Autodesk Inventor part; units mm, degrees
ref_plane "YZ Plane" through (0, 0, 0) normal (1, 0, 0) x (0, 1, 0)
ref_plane "XZ Plane" through (0, 0, 0) normal (0, 1, 0) x (-1, 0, 0)
ref_plane "XY Plane" through (0, 0, 0) normal (0, 0, 1) x (1, 0, 0)
sketch "草圖1" plane through (0, 0, 0) normal (0, 1, 0) x (-1, 0, 0)
  line L0 (0, 0) -> (-20, 0)
  line L1 (-20, 0) -> (-20, -30)
  line L2 (-20, -30) -> (0, -30)
  line L3 (0, -30) -> (0, 0)
  line L4 (-20, -30) -> (-60, -30)
  line L5 (-60, -30) -> (-60, 10)
  line L6 (-60, 10) -> (-20, 10)
  line L7 (-20, 10) -> (-20, -30)
  dimension "d0" = 20
  dimension "d1" = 40
  dimension "d2" = 40
  dimension "d3" = 30
extrude "擠出1" add sketch "草圖1" along normal blind 10
chamfer "倒角1" distance 30 distance2 40 1 edges at (60, 5, 10) measured on face at (33.3333, 3.3333, 10)
sketch "草圖2" plane through (0, 0, -30) normal (-1, 0, 0) x (0, 0, 1)
  line L0 (0, 0) -> (0, 10)
  line L1 (0, 10) -> (20, 10)
  line L2 (20, 10) -> (20, 30)
  line L3 (20, 30) -> (0, 30)
  line L4 (0, 30) -> (0, 10)
  point P0 (30, 0)
  dimension "d9" = 20
  dimension "d10" = 20
extrude "擠出2" add sketch "草圖2" against normal blind 30
chamfer "倒角2" distance 20 distance2 10 1 edges at (15, 30, -10) measured on face at (10, 30, -16.6667)
properties part number "43"
Geometry check sheet. Reference: the model listing, model coordinates, mm. A direction names the side the tool comes from. Give positions to 0.01 mm unless a question says otherwise; leave off trailing zeros. Order: outer loops, then holes, each group sorted by start corner. A loop starts at its lowest first (then second) coordinate and runs counter-clockwise, first axis right, second up. Notation, with made-up numbers: (11, -12.5) - (60, -12.5) arc R24 cw to (60, -2.5) - close; hole circle Ø5 at (-30, 5). An arc over 180 degrees is marked (long way). Answer in a Markdown table with one row per item. Add a question column.
Q1. Gauge pin test, flat ends, axial feed: pin 1 (11 mm diameter, centred on x = 12, y = 15, fed in from +Z); pin 2 (10 mm diameter, centred on x = 9, z = -24.5, fed in from +Y); pin 3 (5 mm diameter, centred on y = 3.5, z = 3.5, fed in from -X). Record the tip position at first contact, or that the pin passes through.
Q2. Cross-section at C-C, the plane z = -25. Enter the section's corners in (x, y), then the cut area to 3 significant figures.
Q3. Tool access check on faces 1 (the flat face through (45, 5, -10)), 2 (the flat face through (30, 18, -20)), 3 (the flat face through (0, 12, -19)), 4 (the flat face through (15, 15, -10)), 5 (the flat face through (10, 5, 0)). Record the directions out of +Z, -Z, +X, -X, +Y, -Y that give a thin tool (end or side, any length) a straight path to the whole face; none if there is none.
Q4. Material ranges on probe 1 along Y at (x, z) = (6, -4); probe 2 along Z at (x, y) = (25, 11); probe 3 along Z at (x, y) = (12, 2), recorded low to high. Write a range as from..to.
Q5. Cross-section at D-D, the plane y = 12.5. Enter the section's corners in (x, z).
Check values:
| question | item | result |
|---|---|---|
| 1 | pin 1 | stops at z = 0 |
| 1 | pin 2 | stops at y = 29.75 |
| 1 | pin 3 | stops at x = 20 |
| 2 | outline | (0, 0) - (56.25, 0) - (56.25, 10) - (30, 10) - (30, 27.5) - (0, 27.5) - close |
| 2 | area | 1,090 mm^2 |
| 3 | face 1 | +Z, +X, +Y, -Y |
| 3 | face 2 | +Z, -Z, +X, +Y |
| 3 | face 3 | +Z, -Z, -X, +Y, -Y |
| 3 | face 4 | +Z, +X, -X, +Y |
| 3 | face 5 | +Z, -X, +Y, -Y |
| 4 | probe 1 | y = 0..10 |
| 4 | probe 2 | z = -30..-10 |
| 4 | probe 3 | z = -30..0 |
| 5 | outline | (0, -30) - (30, -30) - (30, -10) - (0, -10) - close |
